Geometry: final body of the model. Coordinates: model frame, mm. A direction names the side the tool comes from. Give positions to 0.01 mm unless a question says otherwise; leave off trailing zeros. Write each loop counter-clockwise with the first axis right and the second up, starting at its lowest first coordinate (ties: lowest second). Pieces come first, ordered by that corner, then holes.
Autodesk Inventor part; units mm, degrees
ref_plane "YZ Plane" through (0, 0, 0) normal (1, 0, 0) x (0, 1, 0)
ref_plane "XZ Plane" through (0, 0, 0) normal (0, 1, 0) x (-1, 0, 0)
ref_plane "XY Plane" through (0, 0, 0) normal (0, 0, 1) x (1, 0, 0)
sketch "Sketch2" plane through (0, 0, 0) normal (0, 1, 0) x (-1, 0, 0)
  line L0 (-94, 28.5) -> (94, 28.5) construction
  line L1 (94, 28.5) -> (94, -28.5) construction
  line L2 (94, -28.5) -> (-94, -28.5) construction
  line L3 (-94, -28.5) -> (-94, 28.5) construction
  line L4 (-94, 28.5) -> (94, -28.5) construction
  line L5 (94, 28.5) -> (-94, -28.5) construction
  line L6 (78.6703, -31.5) -> (-78.6703, -31.5)
  line L7 (-97, -13.1703) -> (-97, 13.1703)
  line L8 (-78.6703, 31.5) -> (78.6703, 31.5)
  line L9 (97, 13.1703) -> (97, -13.1703)
  arc A0 (89.2832, -34.9615) -> (100.4615, -23.7832) centre (94, -28.5) ccw
  arc A1 (100.4615, 23.7832) -> (89.2832, 34.9615) centre (94, 28.5) ccw
  arc A2 (-89.2832, 34.9615) -> (-100.4615, 23.7832) centre (-94, 28.5) ccw
  arc A3 (-100.4615, -23.7832) -> (-89.2832, -34.9615) centre (-94, -28.5) ccw
  arc A4 (89.2832, -34.9615) -> (78.6703, -31.5) centre (78.6703, -49.5) ccw
  arc A5 (97, -13.1703) -> (100.4615, -23.7832) centre (115, -13.1703) ccw
  arc A6 (100.4615, 23.7832) -> (97, 13.1703) centre (115, 13.1703) ccw
  arc A7 (78.6703, 31.5) -> (89.2832, 34.9615) centre (78.6703, 49.5) ccw
  arc A8 (-89.2832, 34.9615) -> (-78.6703, 31.5) centre (-78.6703, 49.5) ccw
  arc A9 (-97, 13.1703) -> (-100.4615, 23.7832) centre (-115, 13.1703) ccw
  arc A10 (-100.4615, -23.7832) -> (-97, -13.1703) centre (-115, -13.1703) ccw
  arc A11 (-78.6703, -31.5) -> (-89.2832, -34.9615) centre (-78.6703, -49.5) ccw
  circle A12 centre (94, -28.5) radius 1.6
  circle A13 centre (94, 28.5) radius 1.6
  circle A14 centre (-94, -28.5) radius 1.6
  circle A15 centre (-94, 28.5) radius 1.6
  circle A16 centre (94, -28.5) radius 3 construction
  circle A17 centre (94, 28.5) radius 3 construction
  circle A18 centre (-94, 28.5) radius 3 construction
  circle A19 centre (-94, -28.5) radius 3 construction
  point P0 (0, 0)
  point P1 (86.5838, -31.5)
  point P2 (-86.5838, -31.5)
  point P3 (-97, -21.0838)
  point P4 (-97, 21.0838)
  point P5 (-86.5838, 31.5)
  point P6 (86.5838, 31.5)
  point P7 (97, 21.0838)
  point P8 (97, -21.0838)
  dimension "d6" = 3
  dimension "d7" = 3
  dimension "d8" = 3
  dimension "d9" = 3
  dimension "d10" = 8
  dimension "d11" = 18
  dimension "d14" = 3.2
  dimension "d15" = 63
  dimension "d16" = 194
  dimension "d17" = 6
extrude "Extrusion1" add sketch "Sketch2" along normal blind 1.5
sketch "Sketch3" plane through (0, 1.5, 0) normal (0, 1, 0) x (1, 0, 0)
  line L0 (84, -21) -> (-84, -21) construction
  line L1 (-84, -21) -> (-84, 21) construction
  line L2 (-84, 21) -> (84, 21) construction
  line L3 (84, 21) -> (84, -21) construction
  line L4 (84, -21) -> (-84, 21) construction
  line L5 (-84, -21) -> (84, 21) construction
  circle A0 centre (-84, 21) radius 1.6
  circle A1 centre (-84, -21) radius 1.6
  circle A2 centre (84, -21) radius 1.6
  circle A3 centre (84, 21) radius 1.6
  point P0 (0, 0)
  dimension "d18" = 168
  dimension "d19" = 42
  dimension "d20" = 3.2
extrude "Extrusion2" cut sketch "Sketch3" against normal through all
equation "\"d7\" = d6"
equation "\"d8\" = d6"
equation "\"d9\" = d8"
equation "\"d21\" = d20"
properties part number "BaseLayer"
Q1. Pull-direction query (Z, two-part tool) for faces 1 (the cylindrical face through (-97.912, 0.74, -18.827)), 2 (the flat face through (1, 1.5, 1)), 3 (the cylindrical face through (-84.327, 0.74, 32.412)); classes: released by +Z, released by -Z, zero draft, split by the parting line, or undercut.
Filled sheet:
face 1: undercut
face 2: zero draft
face 3: released by +Z
Q2. Access query for faces 4 (the cylindrical face through (-97.863, 0.74, 18.676)), 5 (the cylindrical face through (97.912, 0.74, 18.827)), 6 (the cylindrical face through (-84.176, 0.74, -32.363)), 7 (the cylindrical face through (84.176, 0.74, 32.363)). Directions: +Z, -Z, +X, -X, +Y, -Y. A direction counts if a zero-diameter tool reaches every point of the face in a straight line with its end or side. Return the directions, or none.
Filled sheet:
face 4: -X, +Y, -Y
face 5: +X, +Y, -Y
face 6: -Z, +Y, -Y
face 7: +Z, +Y, -Y
Q3. Ray query, line 1 along Z through (x, y) = (94, 1.2); line 2 along Z through (x, y) = (84, 1.05); line 3 along X through (y, z) = (1.1, 21). Return the intervals inside material, ascending.
Filled sheet:
line 1: z = -36.5 to -30.1, -26.9 to 26.9, 30.1 to 36.5
line 2: z = -32.31 to -22.6, -19.4 to 19.4, 22.6 to 32.31
line 3: x = -98.79 to -85.6, -82.4 to 82.4, 85.6 to 98.79
Q4. Section B-B on x = -45. Output: boundary loops of the cut face in (y, z), plus the area to 3 significant figures.
Filled sheet:
outline: (0, -31.5) - (1.5, -31.5) - (1.5, 31.5) - (0, 31.5) - close
area: 94.5 mm2
Q5. Section C-C on z = -17.5. Output: boundary loops of the cut face in (x, y).
Filled sheet:
outline: (-97.53, 0) - (97.53, 0) - (97.53, 1.5) - (-97.53, 1.5) - close
Q6. Pin query (flat end, axial travel): P1, Ø2.5, axis at x = 94, z = -28.5, coming from the +Y side; P2, Ø0.8, axis at y = 1, z = -0.5, coming from the -X side; P3, Ø0.8, axis at x = -10, y = 0.5, coming from the -Z side. Return the tip coordinate at first contact, or that it passes through.
Filled sheet:
P1: passes through
P2: stops at x = -97
P3: stops at z = -31.5
Q7. Section A-A on y = 1.1. Count the separate pieces of the cut face and the enclosed holes in it, plus the area to 3 significant figures.
Filled sheet:
separate pieces: 1
enclosed holes: 8
area: 12,600 mm2
